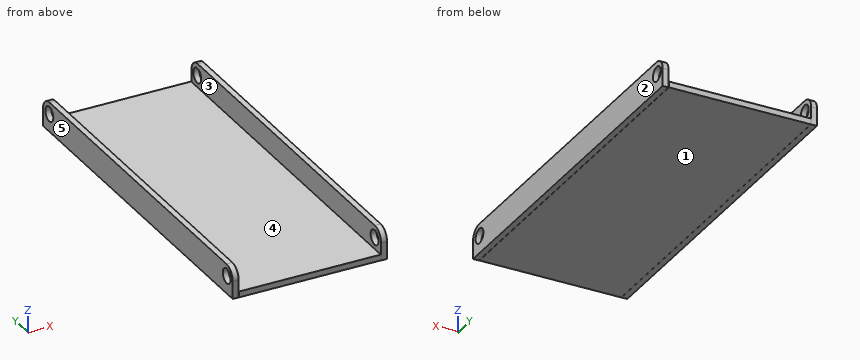
from build123d import *

# Parameters (mm, degrees)
F0_W     = 60.96
F0_H     = 152.4
F1_DEPTH = 2.54
F2_W     = 152.4
F2_H     = 12.7
F3_DEPTH = 2.54
F4_W     = 152.4
F4_H     = 12.7
F5_DEPTH = 2.54
F6_R     = 5.08
F7_R     = 3.175
F8_DEPTH = 90.17


with BuildPart() as f1:
    # F0 (on Top) → F1 (new body)
    with BuildSketch(Plane.XY):
        Rectangle(F0_W, F0_H)
    extrude(amount=F1_DEPTH)

    # F2 (on face) → F3 (join)
    with BuildSketch(Plane.YZ.offset(30.48)):
        with Locations((-0.243933, 6.454543)):
            Rectangle(F2_W, F2_H)
    extrude(amount=F3_DEPTH)

    # F4 (on face) → F5 (join)
    with BuildSketch(Plane(origin=(-30.48, 0, 0), x_dir=(0, -1, 0), z_dir=(-1, 0, 0))):
        with Locations((-0.127775, 6.291921)):
            Rectangle(F4_W, F4_H)
    extrude(amount=F5_DEPTH)

    # F6
    f6_edges = [f1.edges().sort_by_distance(p)[0] for p in [
        (31.75, -76.443933, 12.804543),
        (-31.75, -76.072225, 12.641921),
        (31.75, 75.956067, 12.804543),
        (-31.75, 76.327775, 12.641921),
    ]]
    fillet(f6_edges, radius=F6_R)

    # F7 (on face) → F8 (cut)
    with BuildSketch(Plane(origin=(-33.02, 0, 0), x_dir=(0, -1, 0), z_dir=(-1, 0, 0))):
        with Locations((-71.247775, 7.561921)):
            Circle(F7_R)
        with Locations((71.247775, 7.561921)):
            Circle(F7_R)
    extrude(amount=-F8_DEPTH, mode=Mode.SUBTRACT)


solid = f1.part
Geometry: final body of the model. Coordinates: model frame, mm. Face numbers are marked on the shaded views. A direction names the side the tool comes from. Give positions to 0.01 mm unless a question says otherwise; leave off trailing zeros. Write each loop counter-clockwise with the first axis right and the second up, starting at its lowest first coordinate (ties: lowest second). Pieces come first, ordered by that corner, then holes. Notation, with made-up numbers: (80, 10) -> (96, 10) arc R29 cw to (96, 39) -> close; hole circle Ø9 at (-18.75, -33.75). An arc over 180 degrees is marked (long way). Answer in a Markdown table with one row per item.
(1) Section query A-A on y = 20. Return loops of the section in (x, z).
Answers below:
| item | result |
|---|---|
| outline | (-33.02, -0.06) -> (-30.48, -0.06) -> (-30.48, 0) -> (30.48, 0) -> (30.48, 0.1) -> (33.02, 0.1) -> (33.02, 12.8) -> (30.48, 12.8) -> (30.48, 2.54) -> (-30.48, 2.54) -> (-30.48, 12.64) -> (-33.02, 12.64) -> close |
(2) Ray query, line 1 along X through (y, z) = (59.5, 6.5); line 2 along Z through (x, y) = (-28, 36); line 3 along Y through (x, z) = (-23, 1). Return the intervals inside material, ascending. Write a range as [from, to].
Answers below:
| item | result |
|---|---|
| line 1 | [-33.02, -30.48], [30.48, 33.02] |
| line 2 | [0, 2.54] |
| line 3 | [-76.2, 76.2] |
(3) Set-up query: the marked faces 4 and 5. Return all of +Z, -Z, +X, -X, +Y, -Y with unobstructed straight access to the full face (end or side cutting, diameter ignored); none if empty.
Answers below:
| item | result |
|---|---|
| face 4 | +Z, +Y, -Y |
| face 5 | +Z, -Z, -X, +Y, -Y |
(4) Section query B-B on z = 9.25. Return loops of the section in (x, y).
Answers below:
| item | result |
|---|---|
| outline | (-33.02, -75.78) -> (-30.48, -75.78) -> (-30.48, -73.94) -> (-33.02, -73.94) -> close; (-33.02, -68.56) -> (-30.48, -68.56) -> (-30.48, 68.56) -> (-33.02, 68.56) -> close; (-33.02, 73.94) -> (-30.48, 73.94) -> (-30.48, 76.04) -> (-33.02, 76.04) -> close; (30.48, -76.21) -> (33.02, -76.21) -> (33.02, -73.94) -> (30.48, -73.94) -> close; (30.48, -68.56) -> (33.02, -68.56) -> (33.02, 68.56) -> (30.48, 68.56) -> close; (30.48, 73.94) -> (33.02, 73.94) -> (33.02, 75.72) -> (30.48, 75.72) -> close |
(5) Section query C-C on x = -22. Return loops of the section in (y, z), then the cut area to 3 significant figures.
Answers below:
| item | result |
|---|---|
| outline | (-76.2, 0) -> (76.2, 0) -> (76.2, 2.54) -> (-76.2, 2.54) -> close |
| area | 387 mm^2 |
(6) Pin query (flat end, axial travel): pin 1 (0.8 mm diameter, centred on x = 8, z = 1, fed in from -Y); pin 2 (8 mm diameter, centred on x = -15, y = -30.5, fed in from +Z); pin 3 (4 mm diameter, centred on y = -71.25, z = 7.56, fed in from -X); pin 4 (1.3 mm diameter, centred on x = 31.5, y = 30.5, fed in from -Z). Return the tip coordinate at first contact, or that it passes through.
Answers below:
| item | result |
|---|---|
| pin 1 | y = -76.2 |
| pin 2 | z = 2.54 |
| pin 3 | through |
| pin 4 | z = 0.1 |
(7) Draft query along X for the marked faces 1, 2 and 3. Return one class per face: +X half, -X half, draft (parallel to the pull), parting line (faces both ways), or undercut.
Answers below:
| item | result |
|---|---|
| face 1 | draft |
| face 2 | +X half |
| face 3 | undercut |
